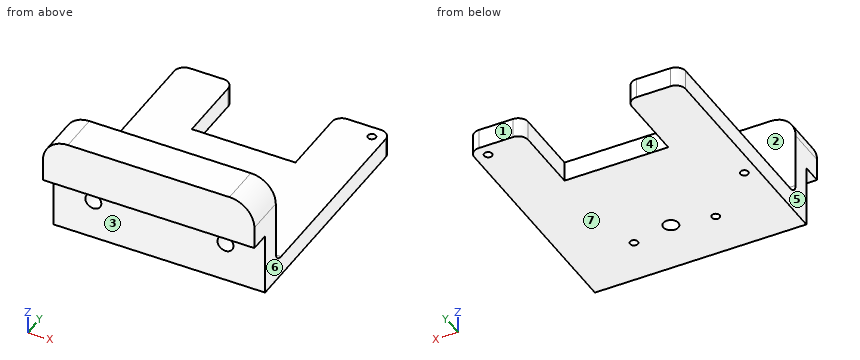
from build123d import *

# Parameters (mm, degrees)
BOSS_EXTRUDE1_DEPTH = 26.924
SKETCH2_R           = 1.0033
SKETCH2_R_2         = 1.905
CUT_EXTRUDE1_DEPTH  = 51.308
SKETCH3_W           = 26.416
SKETCH3_H           = 19.812
CUT_EXTRUDE2_DEPTH  = 5.08
FILLET1_R           = 6.35
FILLET2_R           = 2.54
FILLET3_R           = 2.54
SKETCH4_R           = 2.032
CUT_EXTRUDE3_DEPTH  = 66.185768423


with BuildPart() as part:
    # Sketch1 → Boss-Extrude1 (new, symmetric)
    with BuildSketch(Plane(origin=(0, 0, 0), x_dir=(0, 0, -1), z_dir=(1, 0, 0))):
        Polygon((-10.795, -34.4678), (5.08, -34.4678), (5.08, 25.4), (0, 25.4), (0, -29.3878), (-22.86, -29.3878), (-22.86, -39.5478), (-10.795, -39.5478), align=None)
    extrude(amount=BOSS_EXTRUDE1_DEPTH, both=True)

    # Sketch2 → Cut-Extrude1 (cut)
    with BuildSketch(Plane.XY):
        with Locations((23.749, 22.225)):
            Circle(SKETCH2_R)
        with Locations((-10.414, -22.225)):
            Circle(SKETCH2_R)
        with Locations((10.414, -22.225)):
            Circle(SKETCH2_R)
        with Locations((0, -20.32)):
            Circle(SKETCH2_R_2)
        with Locations((-23.749, -10.922)):
            Circle(SKETCH2_R)
    extrude(amount=-CUT_EXTRUDE1_DEPTH, mode=Mode.SUBTRACT)

    # Sketch3 → Cut-Extrude2 (cut)
    with BuildSketch(Plane.XY):
        with Locations((0, 15.494)):
            Rectangle(SKETCH3_W, SKETCH3_H)
    extrude(amount=-CUT_EXTRUDE2_DEPTH, mode=Mode.SUBTRACT)

    # Fillet1
    fillet1_edges = [part.edges().sort_by_distance(p)[0] for p in [
        (26.924, -34.4678, 22.86),
        (-26.924, -34.4678, 22.86),
    ]]
    fillet(fillet1_edges, radius=FILLET1_R)

    # Fillet2
    fillet2_edges = [part.edges().sort_by_distance(p)[0] for p in [
        (26.924, 25.4, -2.54),
        (-13.208, 25.4, -2.54),
        (13.208, 25.4, -2.54),
        (-26.924, 25.4, -2.54),
    ]]
    fillet(fillet2_edges, radius=FILLET2_R)

    # Fillet3
    fillet3_edges = [part.edges().sort_by_distance(p)[0] for p in [
        (0, -29.3878, 0),
    ]]
    fillet(fillet3_edges, radius=FILLET3_R)

    # Sketch4 → Cut-Extrude3 (cut, through all)
    with BuildSketch(Plane(origin=(0, -29.3878, 0), x_dir=(1, 0, 0), z_dir=(0, 1, 0))):
        with Locations(Location((-16.8275, -5.08, 0), (0, 0, 270))):
            Circle(SKETCH4_R)
        with Locations(Location((16.8275, -5.08, 0), (0, 0, 270))):
            Circle(SKETCH4_R)
    extrude(amount=-CUT_EXTRUDE3_DEPTH, mode=Mode.SUBTRACT)


solid = part.part
Build history of the part. All positions in model axes, mm. Face numbers are marked on the shaded views. A direction names the side the tool comes from. Coordinates: 2 decimals unless noted, no trailing zeros. Write each loop counter-clockwise with the first axis right and the second up, starting at its lowest first coordinate (ties: lowest second). Pieces come first, ordered by that corner, then holes.
(1) Drill centre lines: line 1 (X direction, y = -31.65, z = 5.08); line 2 (Y direction, x = 0, z = -1.5) (3 decimals); line 3 (Y direction, x = -8.5, z = -0.5). Where is each one in solid material? Low to high.
(2) Pin check, flat tips, straight feed: pin 1 Ø6.5 at (x, z) = (16.83, 5.08) entering from -Y; pin 2 Ø5.5 at (x, z) = (6.5, -2) entering from +Y; pin 3 Ø1.2 at (x, y) = (-23.749, -10.922) entering from +Z; pin 4 Ø10 at (x, z) = (7.5, 11.5) entering from +Y. Stop position of each tip, or through.
(3) Cut at A-A on y = -20.32. List the corners of the cut face in (x, z) (3 decimals).
(4) Cut at C-C on x = 0. List the corners of the cut face in (y, z) (3 decimals).
(5) 3-axis set-ups, long thin cutter, end or side, ignore diameter. For the marked faces 1, 2 and 3: which of +Z, -Z, +X, -X, +Y, -Y reach the whole face in a straight line?
(6) Mould opens along X. For the marked faces 4, 5, 6 and 7 say: pulls with the +X half, pulls with the -X half, needs draft (parallel to the pull), parting line crosses it, or undercut.
(7) Cut at D-D on z = 10. List the corners of the cut face in (x, y), and give its area (3 significant figures).
(8) Cut at B-B on z = 5.08. List the corners of the cut face in (x, y), and give its area (3 significant figures).
Working result:
1. line 1: x = -26.92 to -18.86, -14.8 to 14.8, 18.86 to 26.92
1. line 2: y = -34.468 to -22.225, -18.415 to 5.588
1. line 3: y = -34.47 to 5.59
2. pin 1: stops at y = -34.47
2. pin 2: stops at y = 5.59
2. pin 3: passes through
2. pin 4: stops at y = -29.39
3. outline: (-26.924, -5.08) - (-1.905, -5.08) - (-1.905, 0) - (-26.924, 0) - close; (1.905, -5.08) - (26.924, -5.08) - (26.924, 0) - (1.905, 0) - close
4. outline: (-39.548, 10.795) - (-34.468, 10.795) - (-34.468, -5.08) - (-22.225, -5.08) - (-22.225, 0) - (-26.848, 0) arc R2.54 cw to (-29.388, 2.54) - (-29.388, 22.86) - (-39.548, 22.86) - close; (-18.415, -5.08) - (5.588, -5.08) - (5.588, 0) - (-18.415, 0) - close
5. face 1: +Z, -Z, +X, -X, +Y
5. face 2: +Z, +X, -X, +Y
5. face 3: -Z, +X, -X, -Y
6. face 4: undercut
6. face 5: pulls with the -X half
6. face 6: pulls with the +X half
6. face 7: needs draft
7. outline: (-26.92, -34.47) - (26.92, -34.47) - (26.92, -29.39) - (-26.92, -29.39) - close
7. area: 274 mm2
8. outline: (-26.92, -34.47) - (-18.86, -34.47) - (-18.86, -29.39) - (-26.92, -29.39) - close; (-14.8, -34.47) - (14.8, -34.47) - (14.8, -29.39) - (-14.8, -29.39) - close; (18.86, -34.47) - (26.92, -34.47) - (26.92, -29.39) - (18.86, -29.39) - close
8. area: 232 mm2
